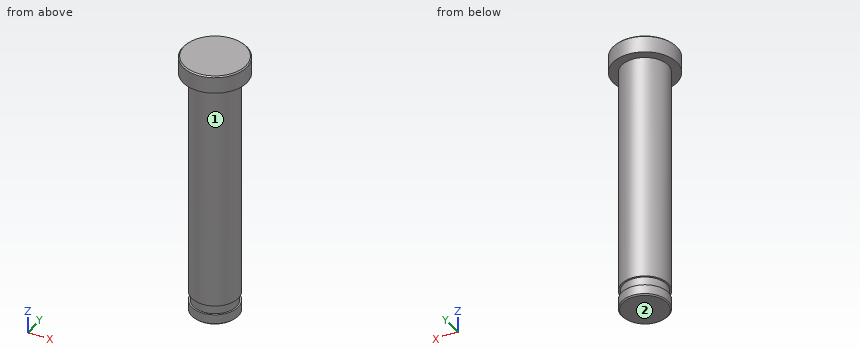
Autodesk Inventor part; units mm, degrees
ref_plane "Work Plane1" through (0, 0, 1.3) normal (0, 0, -1) x (-1, 0, 0)
ref_plane "YZ Plane" through (0, 0, 0) normal (1, 0, 0) x (0, 1, 0)
ref_plane "XZ Plane" through (0, 0, 0) normal (0, 1, 0) x (-1, 0, 0)
sketch "Sketch1" plane through (0, 0, 0) normal (0, 0, 1) x (1, 0, 0)
  circle A0 centre (0, 0) radius 2
  dimension "d0" = 4
extrude "Extrusion1" add sketch "Sketch1" along normal blind 21.5
sketch "Sketch2" plane through (0, 0, 21.5) normal (0, 0, 1) x (1, 0, 0)
  circle A0 centre (0, 0) radius 2.75
  dimension "d3" = 5.5
extrude "Extrusion2" add sketch "Sketch2" along normal blind 1.5
ref_plane "Work Plane1" through (0, 0, 1.3) normal (0, 0, -1) x (-1, 0, 0)
sketch "Sketch3" plane through (0, 0, 1.3) normal (0, 0, -1) x (-1, 0, 0)
  circle A0 centre (0, 0) radius 2
  circle A1 centre (0, 0) radius 1.85
  dimension "d7" = 3.7
extrude "Extrusion3" cut sketch "Sketch3" along normal mid plane 0.8
chamfer "Chamfer1" distance 0.1 angle 45 2 edges at (-2, 0, 0) (-2.75, 0, 23)
properties part number "roller pin" material "Aluminum 3003-H14"
The listing builds one solid part. Answer for the finished solid, in the listing's coordinates (mm). Face numbers are marked on the shaded views. A direction names the side the tool comes from. Give positions to 0.01 mm unless a question says otherwise; leave off trailing zeros. Order: outer loops, then holes, each group sorted by start corner. A loop starts at its lowest first (then second) coordinate and runs counter-clockwise, first axis right, second up. Notation, with made-up numbers: (84, 44) -> (103, 44) arc R34 cw to (103, 81) -> close; hole circle Ø11 at (31.5, 47). An arc over 180 degrees is marked (long way). Answer as CSV lines item,"result". Start each with the question number.
Q1. Find the intervals of material crossed by L1, parallel to Z at x = -1.6, y = 2; L2, parallel to Y at x = 0.35, z = 9.25; L3, parallel to X at y = -1.4, z = 4.75, in increasing order.
Q2. Which of the six approach directions +Z, -Z, +X, -X, +Y, -Y give full straight-line access (tool end or side, diameter ignored) to the marked faces 1 and 2?
Q3. Given pin 1 (1 mm diameter, centred on y = -1.5, z = 9.5, fed in from +X), flat-ended and moving along its own axis, determine where the tip first touches the part or whether it passes through.
Q4. A cutting plane is placed at C-C (z = 16.75). Determine the outline of the cut face in (x, y), then the cut area to 3 significant figures.
Q5. A cutting plane is placed at A-A (x = 0). Determine the outline of the cut face in (y, z), then the cut area to 3 significant figures.
Results found:
1,L1,"21.5 to 23"
1,L2,"-1.97 to 1.97"
1,L3,"-1.43 to 1.43"
2,face 1,"-Z"
2,face 2,"-Z, +X, -X, +Y, -Y"
3,pin 1,"x = 1.73"
4,outline,"circle Ø4 at (0, 0)"
4,area,"12.6 mm2"
5,outline,"(-2.75, 21.5) -> (-2, 21.5) -> (-2, 1.7) -> (-1.85, 1.7) -> (-1.85, 0.9) -> (-2, 0.9) -> (-2, 0.1) -> (-1.9, 0) -> (1.9, 0) -> (2, 0.1) -> (2, 0.9) -> (1.85, 0.9) -> (1.85, 1.7) -> (2, 1.7) -> (2, 21.5) -> (2.75, 21.5) -> (2.75, 22.9) -> (2.65, 23) -> (-2.65, 23) -> (-2.75, 22.9) -> close"
5,area,"94.0 mm2"
